from build123d import *

# Parameters (mm, degrees)
FILLET1_R      = 0.79375
CHAMFER1_SIZE  = 0.79375
CHAMFER1_SIZE2 = 1.374815329


with BuildPart() as part:
    # Sketch1 → Revolve1 (revolve)
    with BuildSketch(Plane.XY):
        Polygon((0, 0), (-9.398, 0), (-9.398, 1.5875), (-6.223, 4.445), (-6.223, 7.62), (-9.398, 7.62), (-9.398, 12.7), (0, 12.7), align=None)
    revolve(axis=Axis((0, 0, 0), (0, 1, 0)))

    # Fillet1
    fillet1_edges = [part.edges().sort_by_distance(p)[0] for p in [
        (9.398, 0, 0),
    ]]
    fillet(fillet1_edges, radius=FILLET1_R)

    # Chamfer1
    chamfer1_edges = [part.edges().sort_by_distance(p)[0] for p in [
        (9.398, 12.7, 0),
    ]]
    chamfer1_side = [part.faces().sort_by_distance(p)[0] for p in [
        (0, 12.7, 0),
    ]]
    chamfer(chamfer1_edges, length=CHAMFER1_SIZE, length2=CHAMFER1_SIZE2, reference=chamfer1_side[0])


solid = part.part
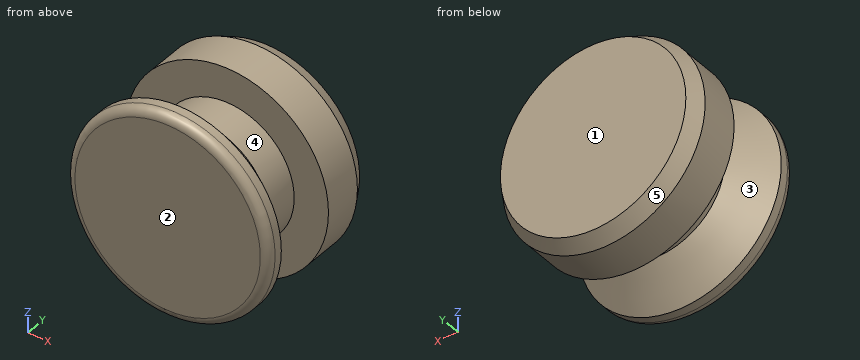
Design review of the part built by this model. Coordinates are the model's own, in mm. Face numbers are marked on the shaded views. A direction names the side the tool comes from. Round coordinates to 2 decimals unless told otherwise and drop trailing zeros. Write each loop counter-clockwise with the first axis right and the second up, starting at its lowest first coordinate (ties: lowest second). Pieces come first, ordered by that corner, then holes. Notation, with made-up numbers: (-21.75, 57.25) - (0.25, 57.25) arc R24 cw to (0.25, 76.25) - close; hole circle Ø3 at (85.5, 40.25). An arc over 180 degrees is marked (long way). Return JSON: item names as keys, results as strings. Group by question number.
Item 1: We need section A-A on x = 0. Write out the cut boundary in (y, z) (1 decimal), and give its area (3 significant figures).
Item 2: We need section D-D on y = 8. Write out the cut boundary in (x, z), and give its area (3 significant figures).
Item 3: Machinability: for the marked faces 4 and 5, which of the approach directions +Z, -Z, +X, -X, +Y, -Y give a long, thin tool a straight path to every point of the face, cutting with its end or side? Answer none if there is none.
Item 4: We need section C-C on y = 6.25. Write out the cut boundary in (x, z).
Item 5: The part is to be moulded in two halves that separate along Y. For the marked faces 1, 2 and 3, say which applies: pulls with the +Y half, pulls with the -Y half, needs draft (parallel to the pull), parting line crosses it, or undercut.
Item 6: Insertion check: P1, Ø5.5, axis at x = -2.5, z = 0.5, coming from the -Y side; P2, Ø5, axis at y = 3, z = 2.5, coming from the +X side; P3, Ø1, axis at x = 0, y = 7, coming from the -Z side; P4, Ø1.5, axis at y = 1.5, z = 4, coming from the -X side. Each pin has a flat end and moves straight along its axis. Give the tip position at first contact, or say it passes through.
Item 7: We need section B-B on z = 0. Write out the cut boundary in (x, y) (1 decimal), and give its area (3 significant figures).
Item 8: For probe 1 along Y at (x, z) = (6.5, -2.5); probe 2 along Y at (x, z) = (-4.5, -8); probe 3 along Z at (x, y) = (8.5, 8), list the stretches that pass through material, from the lowest coordinate up. Write a range as [from, to].
Model answer:
{
 "1": {"outline": "(0, -8.6) arc R0.8 ccw to (0.8, -9.4) - (1.6, -9.4) - (4.4, -6.2) - (7.6, -6.2) - (7.6, -9.4) - (11.3, -9.4) - (12.7, -8.6) - (12.7, 8.6) - (11.3, 9.4) - (7.6, 9.4) - (7.6, 6.2) - (4.4, 6.2) - (1.6, 9.4) - (0.8, 9.4) arc R0.8 ccw to (0, 8.6) - close", "area": "208 mm²"},
 "2": {"outline": "circle Ø18.8 at (0, 0)", "area": "277 mm²"},
 "3": {"face 4": "none", "face 5": "+Y"},
 "4": {"outline": "circle Ø12.45 at (0, 0)"},
 "5": {"face 1": "pulls with the +Y half", "face 2": "pulls with the -Y half", "face 3": "undercut"},
 "6": {"P1": "stops at y = 0", "P2": "stops at x = 9.39", "P3": "stops at z = -6.22", "P4": "stops at x = -8.82"},
 "7": {"outline": "(-9.4, 0.8) arc R0.8 ccw to (-8.6, 0) - (8.6, 0) arc R0.8 ccw to (9.4, 0.8) - (9.4, 1.6) - (6.2, 4.4) - (6.2, 7.6) - (9.4, 7.6) - (9.4, 11.3) - (8.6, 12.7) - (-8.6, 12.7) - (-9.4, 11.3) - (-9.4, 7.6) - (-6.2, 7.6) - (-6.2, 4.4) - (-9.4, 1.6) - close", "area": "208 mm²"},
 "8": {"probe 1": "y = [0, 3.78], [7.62, 12.7]", "probe 2": "y = [0.25, 1.78], [7.62, 11.7]", "probe 3": "z = [-4.01, 4.01]"}
}
